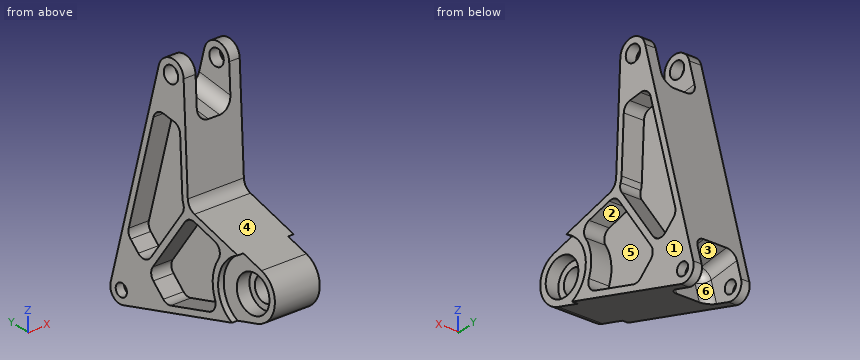
```python
from build123d import *

# Parameters (mm, degrees)
SKETCH1_R               = 3.263900000000121
SKETCH1_R_2             = 4.199999999999976
BOSS_EXTRUDE1_DEPTH     = 15.875
FILLET7_R               = 6.35
CUT_EXTRUDE6_DEPTH      = 25.4
FILLET8_R               = 6.35
CUT_EXTRUDE8_DEPTH      = 20.32
CUT_EXTRUDE9_DEPTH      = 906.5663752758251
CUT_EXTRUDE9_DEPTH_BACK = 3.175
CUT_EXTRUDE10_DEPTH     = 11.43
SKETCH29_R              = 6.349999999999941
CUT_EXTRUDE11_DEPTH     = 906.4543212392226
SKETCH30_R              = 9.525000000000018
CUT_EXTRUDE12_DEPTH     = 7.14375
FILLET10_R              = 4.7625
FILLET10_OF_MIRROR9_R   = 4.7625
SKETCH33_R              = 17.144999999999648
CUT_EXTRUDE14_DEPTH     = 3.175
FILLET11_R              = 4.7625


with BuildPart() as part:
    # Sketch1 → Boss-Extrude1 (new, symmetric)
    with BuildSketch(Plane(origin=(-803.6566332789141, -58.26345281012812, 68.82567852426239), x_dir=(-0.08515417095162939, -0.00241614660156225, -0.9963648575723355), z_dir=(0.9937636896807375, 0.07204582335356381, -0.08510657089457987))):
        with BuildLine():
            ThreePointArc((-664.2038450226969, 436.8184776127322), (-651.8745198787159, 427.9178662715624), (-639.8468613838354, 437.2220896073974))
            Line((-639.8468613838348, 437.2220896073972), (-619.5515204929051, 510.40226291213133))
            ThreePointArc((-619.5515204929051, 510.40226291213133), (-620.9838530756886, 516.4455246988489), (-626.8562553144544, 518.4672768094307))
            Line((-626.8562553144544, 518.4672768094307), (-733.0342996841451, 500.0570320892499))
            ThreePointArc((-733.0342996841451, 500.05703208924996), (-739.1483230926673, 492.6676503574812), (-732.7916358037484, 485.48595339028384))
            Line((-732.7916358037484, 485.4859533902838), (-677.0205822251494, 477.71877799538424))
            Line((-677.0205822251494, 477.71877799538424), (-664.2038450226976, 436.81847761273195))
        make_face()
        with Locations(Location((-625.7562257117465, 512.1230378414245, 0), (0, 0, 0.138795824))):
            Circle(SKETCH1_R, mode=Mode.SUBTRACT)
        with Locations(Location((-731.7743456050367, 492.79045512904787, 0), (0, 0, 0.138795824))):
            Circle(SKETCH1_R_2, mode=Mode.SUBTRACT)
    extrude(amount=BOSS_EXTRUDE1_DEPTH, both=True)

    # Fillet7
    fillet7_edges = [part.edges().sort_by_distance(p)[0] for p in [
        (-780.3962698306742, 419.8482713749311, 745.1689599242694),
    ]]
    fillet(fillet7_edges, radius=FILLET7_R)

    # Sketch23 → Cut-Extrude6 (cut)
    with BuildSketch(Plane(origin=(61.972947811989165, -108.2363846344534, 632.0133130126799), x_dir=(0.9953619214294605, 0.016238085990304504, -0.09482072522199067), z_dir=(0.09620106739496219, -0.16801614414720037, 0.9810789621319872))):
        Polygon((-851.4974580179244, 570.6197226277428), (-849.4828619685262, 535.112578894877), (-830.4634507696352, 536.1916978167321), (-832.4780468190336, 571.698841549598), align=None)
    extrude(amount=-CUT_EXTRUDE6_DEPTH, mode=Mode.SUBTRACT)

    # Fillet8
    fillet8_edges = [part.edges().sort_by_distance(p)[0] for p in [
        (-768.4981336258412, 435.7374633830816, 780.7155057686616),
        (-787.4293319142591, 434.3649904481962, 782.3367859442033),
    ]]
    fillet(fillet8_edges, radius=FILLET8_R)

    # Sketch26 → Cut-Extrude8 (cut)
    with BuildSketch(Plane(origin=(50.277187193507835, -87.80961957666034, 512.7374567291475), x_dir=(-0.9953619214296225, -0.01623864853432569, 0.09482062888268945), z_dir=(-0.0962010673949623, 0.16801614414720273, -0.9810789621319869))):
        Polygon((831.6096354550859, 577.9339524783938), (830.1087716603103, 551.4810443146557), (852.3995223072293, 550.2163296603253), (853.9003861020049, 576.6692378240637), align=None)
    extrude(amount=-CUT_EXTRUDE8_DEPTH, mode=Mode.SUBTRACT)

    # Sketch27 → Cut-Extrude9 (cut, two sides: drawn at the far end of the back side and taken through both)
    with BuildSketch(Plane(origin=(-819.4326318525958, -59.40718025586634, 70.17674533721406), x_dir=(0.08488379068765259, 0.006153900220914947, 0.9963718540738522), z_dir=(-0.9937636896807374, -0.07204582335356426, 0.08510657089458012)).offset(-CUT_EXTRUDE9_DEPTH_BACK)):
        with BuildLine():
            Line((519.6219025840122, 211.91880941976535), (638.4443725730704, 445.9315686732567))
            ThreePointArc((638.4443725730704, 445.9315686732567), (654.0798834896251, 455.31078922151056), (669.3214837157453, 445.3041613048935))
            Line((669.3214837157453, 445.3041613048935), (778.5397566596026, 206.65772885116039))
            Line((778.5397566596026, 206.65772885116039), (767.8761958936219, -318.1367946937436))
            Line((767.8761958936219, -318.1367946937436), (508.95834181803144, -312.87571412513864))
            Line((508.95834181803144, -312.87571412513864), (519.6219025840122, 211.91880941976535))
        make_face()
    extrude(amount=CUT_EXTRUDE9_DEPTH + CUT_EXTRUDE9_DEPTH_BACK, mode=Mode.SUBTRACT)

    # Sketch28 → Cut-Extrude10 (cut)
    with BuildSketch(Plane(origin=(-819.4326318525959, -59.40718025586635, 70.17674533721406), x_dir=(0.08488379068765257, 0.006153900220914946, 0.9963718540738522), z_dir=(-0.9937636896807375, -0.07204582335356424, 0.08510657089458012))):
        with BuildLine():
            Line((641.610435680991, 494.9044603779857), (631.4071387526498, 483.7236998843152))
            Line((631.4071387526498, 483.7236998843152), (639.8115098751724, 452.97250675062605))
            ThreePointArc((639.8115098751724, 452.97250675062605), (654.1443845784224, 458.48513397429696), (668.241493429274, 452.3948237840471))
            Line((668.2414934292741, 452.39482378404716), (674.5635114397776, 472.307585723845))
            ThreePointArc((674.5635114397776, 472.307585723845), (674.9689897543286, 473.36298990652836), (675.4966669350005, 474.3629136263164))
            Line((675.4966669350005, 474.3629136263164), (641.6104356809909, 494.90446037798574))
        make_face()
        with BuildLine():
            Line((653.9539402363619, 508.43045781346063), (643.7918856391113, 497.29489061656125))
            Line((643.7918856391113, 497.2948906165613), (677.6083716229516, 476.79562285771186))
            ThreePointArc((677.6083716229516, 476.79562285771186), (679.842443438827, 478.15968717889757), (682.3634605019174, 478.8641169613652))
            Line((682.3634605019174, 478.8641169613652), (713.0233309253331, 483.01701779228154))
            Line((713.0233309253331, 483.0170177922816), (715.5913760089414, 497.50503494976147))
            Line((715.5913760089414, 497.50503494976147), (653.9539402363619, 508.4304578134607))
        make_face()
    cut_extrude10 = extrude(amount=-CUT_EXTRUDE10_DEPTH, mode=Mode.SUBTRACT)

    # Sketch29 → Cut-Extrude11 (cut, through all)
    with BuildSketch(Plane(origin=(-816.2774321378597, -59.1784347667188, 69.90653197462377), x_dir=(0.08488379068765259, 0.006153900220914947, 0.9963718540738522), z_dir=(-0.9937636896807374, -0.07204582335356423, 0.08510657089458012))):
        with Locations(Location((653.7315776101187, 438.16932755646275, 0), (0, 0, 359.646486586))):
            Circle(SKETCH29_R)
    extrude(amount=-CUT_EXTRUDE11_DEPTH, mode=Mode.SUBTRACT)

    # Sketch30 → Cut-Extrude12 (cut)
    with BuildSketch(Plane(origin=(-816.2774321378599, -59.178434766718816, 69.90653197462377), x_dir=(0.08488379068765257, 0.006153900220914946, 0.9963718540738522), z_dir=(-0.9937636896807375, -0.07204582335356424, 0.08510657089458012))):
        with Locations(Location((653.7315776101187, 438.16932755646275, 0), (0, 0, 359.646486586))):
            Circle(SKETCH30_R)
    cut_extrude12 = extrude(amount=-CUT_EXTRUDE12_DEPTH, mode=Mode.SUBTRACT)

    # Fillet10
    fillet10_edges = [part.edges().sort_by_distance(p)[0] for p in [
        (-788.1552248280682, 427.1450787260482, 780.1267395165396),
        (-788.9848414044336, 441.61097464981503, 782.6854673578397),
        (-795.0068579123044, 452.1284878234392, 721.2716611967566),
        (-795.0642591647301, 440.95953350372866, 711.1464760164944),
        (-790.7115231509628, 420.72202917254344, 744.8402708544758),
        (-789.7422422016995, 396.3274603010962, 735.5073770617572),
        (-792.1972581719219, 396.7286758070525, 707.180541636668),
        (-790.7148679020396, 418.2826927308667, 742.7362277392854),
        (-795.0765812752346, 438.5619361773402, 708.9729406771527),
        (-795.1342154885674, 427.347653060428, 698.8066627989953),
    ]]
    fillet(fillet10_edges, radius=FILLET10_R)

    # Mirror9: Cut-Extrude10, Cut-Extrude12 across plane
    add(cut_extrude10.mirror(Plane(origin=(-803.6566332789141, -58.26345281012812, 68.82567852426239), x_dir=(0.08488379068765235, 0.00615390022091489, 0.9963718540738523), z_dir=(0.9937636896807375, 0.07204582335356381, -0.08510657089457987))), mode=Mode.SUBTRACT)
    add(cut_extrude12.mirror(Plane(origin=(-803.6566332789141, -58.26345281012812, 68.82567852426239), x_dir=(0.08488379068765235, 0.00615390022091489, 0.9963718540738523), z_dir=(0.9937636896807375, 0.07204582335356381, -0.08510657089457987))), mode=Mode.SUBTRACT)

    # Fillet10 of Mirror9
    fillet10_of_mirror9_edges = [part.edges().sort_by_distance(p)[0] for p in [
        (-767.9619466537554, 428.60904985659255, 778.3973739959619),
        (-768.7915632301208, 443.0749457803594, 780.9561018372618),
        (-774.8135797379914, 453.59245895398357, 719.5422956761787),
        (-774.870980990417, 442.4235046342731, 709.4171104959165),
        (-770.5182449766497, 422.18600030308784, 743.1109053338979),
        (-769.5489640273865, 397.79143143164066, 733.7780115411794),
        (-772.0039799976088, 398.192646937597, 705.4511761160901),
        (-770.5215897277267, 419.74666386141104, 741.0068622187075),
        (-774.8833031009216, 440.02590730788467, 707.2435751565748),
        (-774.9409373142544, 428.8116241909724, 697.0772972784174),
    ]]
    fillet(fillet10_of_mirror9_edges, radius=FILLET10_OF_MIRROR9_R)

    # Sketch33 → Cut-Extrude14 (cut)
    with BuildSketch(Plane(origin=(-787.8806347052326, -57.119725364390696, 67.47461171131114), x_dir=(-0.08488379068765259, -0.006153900220914947, -0.9963718540738522), z_dir=(0.9937636896807374, 0.07204582335356423, -0.08510657089458012))):
        with Locations((-653.7315776101188, 438.1693275564627)):
            Circle(SKETCH33_R)
    extrude(amount=-CUT_EXTRUDE14_DEPTH, mode=Mode.SUBTRACT)

    # Fillet11
    fillet11_edges = [part.edges().sort_by_distance(p)[0] for p in [
        (-796.9082546128618, 438.46793345177383, 699.2942172907788),
        (-785.1203512694295, 438.0597382877858, 705.4239621272485),
        (-796.7868884418211, 447.2442527490892, 708.1408484710828),
        (-774.5995240477952, 448.852791028775, 706.240708105348),
        (-774.720890218836, 440.07647173145955, 697.3940769250439),
    ]]
    fillet(fillet11_edges, radius=FILLET11_R)


solid = part.part
```
The model under review builds one solid part; all positions refer to its coordinate system, in mm. Face numbers are marked on the shaded views. A direction names the side the tool comes from. Round coordinates to 2 decimals unless told otherwise and drop trailing zeros. Loops run counter-clockwise (first coordinate to the right, second up) from the corner with the lowest first, then second, coordinate; pieces in that order, holes last. Notation, with made-up numbers: (88, 30) - (108, 30) arc R8 cw to (108, 44) - close; hole circle Ø6 at (-33, -24). An arc over 180 degrees is marked (long way). Use a Markdown table: item, result. Add a question column.
Q1. For probe 1 along Z at (x, y) = (-791, 431.5); probe 2 along X at (y, z) = (427, 757); probe 3 along Z at (x, y) = (-788, 390), list the stretches that pass through material, from the lowest coordinate up.
Q2. Insertion check: pin 1 Ø10 at (x, y) = (-782.5, 418.5) entering from -Z; pin 2 Ø6 at (x, y) = (-768.5, 381.5) entering from +Z; pin 3 Ø1 at (x, y) = (-782, 410.5) entering from -Z. Each pin has a flat end and moves straight along its axis. Give the tip position at first contact, or say it passes through.
Q3. Add section A-A (z = 753). State the section outline as (x, y) points, plus the area to 3 significant figures.
Q4. Machinability: for the marked faces 1, 2 and 3, which of the approach directions +Z, -Z, +X, -X, +Y, -Y give a long, thin tool a straight path to every point of the face, cutting with its end or side? Answer none if there is none.
Q5. The part is to be moulded in two halves that separate along Y. For the marked faces 4, 5 and 6, say which applies: pulls with the +Y half, pulls with the -Y half, needs draft (parallel to the pull), parting line crosses it, or undercut.
Worked answers:
| question | item | result |
|---|---|---|
| 1 | probe 1 | 694.07 to 701.95, 720.82 to 726.97, 781.15 to 797.61, 804.41 to 807.98 |
| 1 | probe 2 | -784.37 to -775.43 |
| 1 | probe 3 | 705.49 to 715.33, 726.34 to 736.69 |
| 2 | pin 1 | z = 695.72 |
| 2 | pin 2 | z = 732.92 |
| 2 | pin 3 | z = 699.21 |
| 3 | outline | (-797.86, 449.58) - (-797.62, 446.37) - (-786.17, 447.02) - (-784.48, 423.78) - (-795.92, 422.82) - (-795.68, 419.62) - (-763.93, 422.29) - (-764.16, 425.49) - (-775.59, 424.53) - (-777.26, 447.53) - (-765.81, 448.19) - (-766.04, 451.41) - close |
| 3 | area | 412 mm² |
| 4 | face 1 | -Z, +X, +Y |
| 4 | face 2 | none |
| 4 | face 3 | -Z, +Y |
| 5 | face 4 | pulls with the -Y half |
| 5 | face 5 | undercut |
| 5 | face 6 | pulls with the +Y half |
